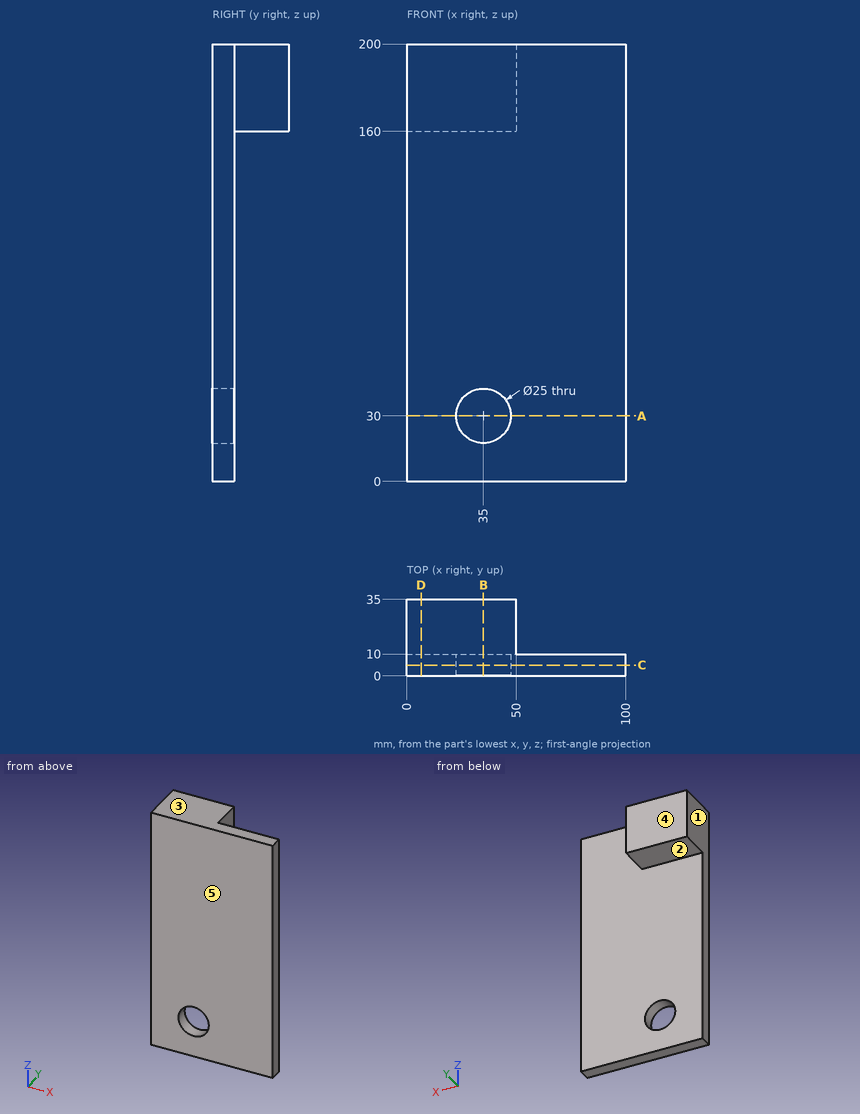
Verification items for this drawing (mm, ordinates from the low corner). A direction names the side the tool comes from. Round coordinates to 2 decimals unless told otherwise and drop trailing zeros. Order: outer loops, then holes, each group sorted by start corner. A loop starts at its lowest first (then second) coordinate and runs counter-clockwise, first axis right, second up.
1) Depth check by flat-ended pin: pin 1 (1.5 mm diameter, centred on x = 15.5, z = 113.5, fed in from +Y); pin 2 (20 mm diameter, centred on x = 14, y = 24.5, fed in from -Z); pin 3 (7.5 mm diameter, centred on y = 26, z = 175, fed in from +X). Enter the tip coordinate at first touch or a pass-through.
Geometry says:
pin 1: stops at y = 10
pin 2: stops at z = 160
pin 3: stops at x = 50
2) Material ranges on line 1 (Z direction, x = 35, y = 7.5); line 2 (X direction, y = 4, z = 30); line 3 (Y direction, x = 41.5, z = 65), recorded low to high.
Geometry says:
line 1: z = 0 to 17.5, 42.5 to 200
line 2: x = 0 to 22.5, 47.5 to 100
line 3: y = 0 to 10
3) Cross-section at B-B, the plane x = 35. Record the cut outline in (y, z).
Geometry says:
outline: (0, 0) - (10, 0) - (10, 17.5) - (0, 17.5) - close; (0, 42.5) - (10, 42.5) - (10, 160) - (35, 160) - (35, 200) - (0, 200) - close
4) Cross-section at A-A, the plane z = 30. Record the cut outline in (x, y).
Geometry says:
outline: (0, 0) - (22.5, 0) - (22.5, 10) - (0, 10) - close; (47.5, 0) - (100, 0) - (100, 10) - (47.5, 10) - close
5) Cross-section at D-D, the plane x = 6.5. Record the cut outline in (y, z), plus the area to 3 significant figures.
Geometry says:
outline: (0, 0) - (10, 0) - (10, 160) - (35, 160) - (35, 200) - (0, 200) - close
area: 3,000 mm2
6) Tool access check on the marked faces 1 and 2. Record the directions out of +Z, -Z, +X, -X, +Y, -Y that give a thin tool (end or side, any length) a straight path to the whole face; none if there is none.
Geometry says:
face 1: +Z, -Z, -X, +Y, -Y
face 2: -Z, +X, -X, +Y
7) Cross-section at C-C, the plane y = 5. Record the cut outline in (x, z), plus the area to 3 significant figures.
Geometry says:
outline: (0, 0) - (100, 0) - (100, 200) - (0, 200) - close; hole circle Ø25 at (35, 30)
area: 19,500 mm2
8) Draft check along Y on the marked faces 3, 4 and 5. Enter one of: +Y half, -Y half, draft (parallel to the pull), parting line (faces both ways), or undercut.
Geometry says:
face 3: draft
face 4: +Y half
face 5: -Y half
